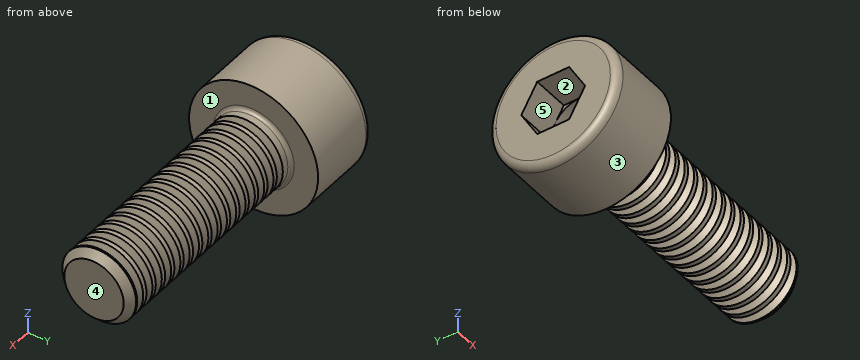
```python
from build123d import *

# Parameters (mm, degrees)
BASEHEADSKE_R   = 3.5
BASEHEAD_DEPTH  = 4
CUTSOCKET_DEPTH = 2
FILLET1_R       = 0.2
FILLET2_R       = 0.4
THDSCHPAT_COUNT = 16
THDSCHPAT_PITCH = 0.7


with BuildPart() as part:
    # BaseHeadSke → BaseHead (new body)
    with BuildSketch(Plane(origin=(0, 0, 0), x_dir=(0, 0, -1), z_dir=(1, 0, 0))):
        Circle(BASEHEADSKE_R)
    extrude(amount=BASEHEAD_DEPTH)

    # BodySke → BaseBody (revolve)
    with BuildSketch(Plane.XY):
        Polygon((0, 0), (16, 0), (16, 1.61), (15.61, 2), (0, 2), align=None)
    revolve(axis=Axis((0, 0, 0), (1, 0, 0)))

    # CutSocketSke → CutSocket (cut)
    with BuildSketch(Plane(origin=(0, 0, 0), x_dir=(0, 0, -1), z_dir=(1, 0, 0))):
        Polygon((0, 1.732050808), (-1.5, 0.866025404), (-1.5, -0.866025404), (0, -1.732050808), (1.5, -0.866025404), (1.5, 0.866025404), align=None)
    extrude(amount=CUTSOCKET_DEPTH, mode=Mode.SUBTRACT)

    # CutHoleSke → CutHole (revolve, cut)
    with BuildSketch(Plane.XY):
        Polygon((0, 1.5), (2.6, 1.5), (3.466025404, 0), (0, 0), align=None)
    revolve(axis=Axis((0, 0, 0), (1, 0, 0)), mode=Mode.SUBTRACT)

    # Fillet1
    fillet1_edges = [part.edges().sort_by_distance(p)[0] for p in [
        (4, -2, 0),
    ]]
    fillet(fillet1_edges, radius=FILLET1_R)

    # Fillet2
    fillet2_edges = [part.edges().sort_by_distance(p)[0] for p in [
        (0, 0, 3.5),
    ]]
    fillet(fillet2_edges, radius=FILLET2_R)

    # ThdSchSke → ThreadSchematic (revolve, cut)
    with BuildSketch(Plane.XY):
        Polygon((15.074833395, 2.45033321), (15.074833395, 2), (15.3, 1.61), (15.525166605, 2), (15.525166605, 2.45033321), align=None)
    threadschematic = revolve(axis=Axis((0, 0, 0), (1, 0, 0)), mode=Mode.SUBTRACT)

    # ThdSchPat: ThreadSchematic ×16
    with Locations(*[(-i * THDSCHPAT_PITCH, 0, 0) for i in range(1, THDSCHPAT_COUNT)]):
        add(threadschematic, mode=Mode.SUBTRACT)


solid = part.part
```
Read the model definition and answer for the solid it produces. Units are mm, in the model's axes. Face numbers are marked on the shaded views. A direction names the side the tool comes from. Coordinates: 2 decimals unless noted, no trailing zeros. Loops run counter-clockwise (first coordinate to the right, second up) from the corner with the lowest first, then second, coordinate; pieces in that order, holes last.
(1) The part is cut by section A-A (x = 1.75). Determine the outline of the cut face in (y, z), and give its area (3 significant figures).
Solution:
outline: circle Ø7 at (0, 0); hole (-1.73, 0) - (-0.87, -1.5) - (0.87, -1.5) - (1.73, 0) - (0.87, 1.5) - (-0.87, 1.5) - close
area: 30.7 mm2
(2) The mould has two halves that part along Z. Classify the marked faces 1, 2 and 3: released by +Z, released by -Z, zero draft, split by the parting line, or undercut.
Solution:
face 1: zero draft
face 2: undercut
face 3: split by the parting line
(3) Flat-ended cylindrical pins translate along their axes: pin 1 Ø3 at (x, z) = (9.5, 2.5) entering from -Y; pin 2 Ø1.5 at (y, z) = (0.5, 0.5) entering from -X. Find the tip coordinate at first contact, or state that the pin passes through.
Solution:
pin 1: stops at y = -1.73
pin 2: stops at x = 2.62
(4) A tool of negligible diameter and unlimited length cuts with its end or side. For the marked faces 4 and 5, from which of +Z, -Z, +X, -X, +Y, -Y can it reach the whole face along a straight path? Write none if from no direction.
Solution:
face 4: +Z, -Z, +X, +Y, -Y
face 5: -X
(5) Consider line 1 along Y through (x, z) = (2.4, 0); line 2 along X through (y, z) = (2.5, -0.5); line 3 along X through (y, z) = (0.25, -1). Determine where each line is inside the solid, lowest interval first.
Solution:
line 1: y = -3.5 to -1.5, 1.5 to 3.5
line 2: x = 0 to 4
line 3: x = 2.87 to 16
